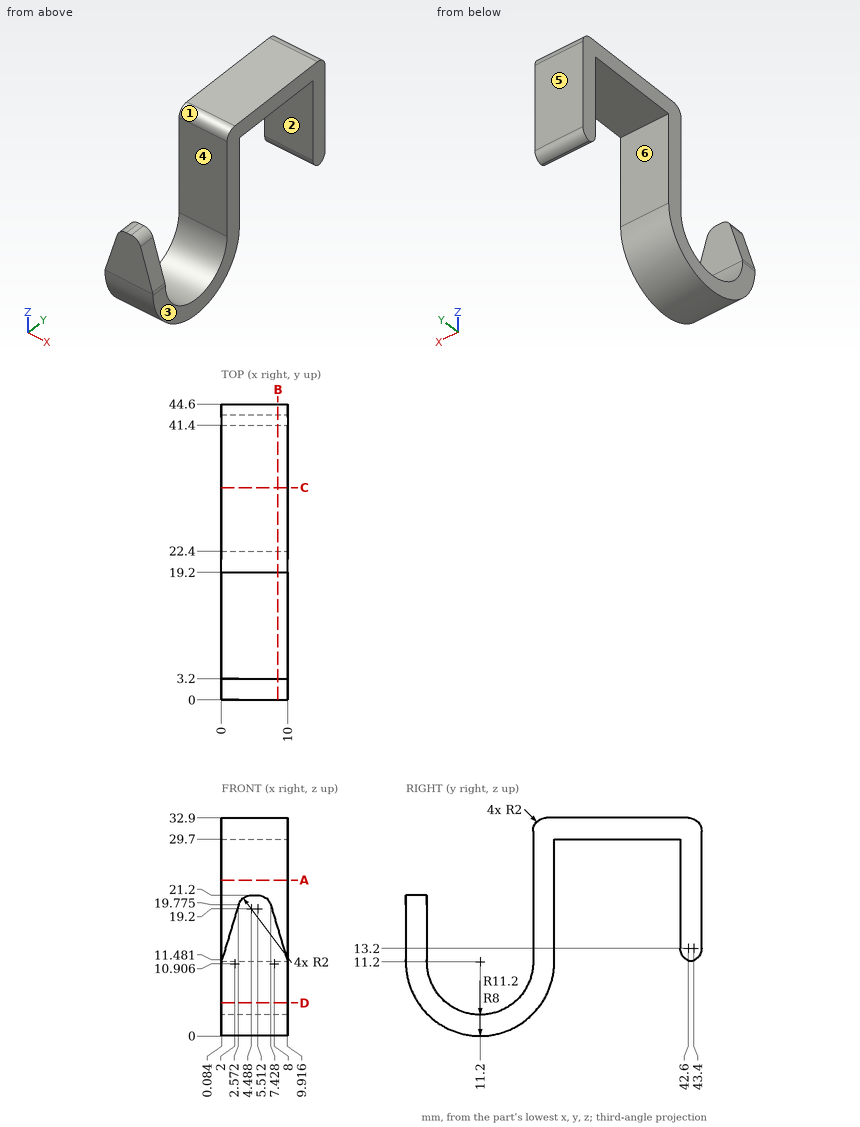
Part print with two shaded views. Sizes in mm from the minimum x, y, z corner. A direction names the side the tool comes from. Round coordinates to 2 decimals unless told otherwise and drop trailing zeros. Write each loop counter-clockwise with the first axis right and the second up, starting at its lowest first coordinate (ties: lowest second). Pieces come first, ordered by that corner, then holes. Notation, with made-up numbers: M -20,28 L -9,28 A27 cw -9,65 Z; hole C 49,67.5 d2. An arc over 180 degrees is marked long. Answer as CSV lines item,"result". Start each with the question number.
1) Drill centre lines: L1, parallel to Y at x = 4.5, z = 19; L2, parallel to Y at x = 1, z = 25.5; L3, parallel to Y at x = 9, z = 12. Where is each one in solid material? Low to high.
2) Band-saw the part on D-D (z = 5). List the corners of the cut face in (x, y) (1 decimal).
3) Band-saw the part on B-B (x = 8.5). List the corners of the cut face in (y, z).
4) Drop flat-ended pins along their axis: pin 1 (3 mm diameter, centred on x = 1.5, y = 6, fed in from -Z); pin 2 (2 mm diameter, centred on x = 4, y = 8, fed in from -Z); pin 3 (5 mm diameter, centred on x = 5.5, y = 9, fed in from +Z) (1 decimal). Give the stop position or say it passes through.
5) Which spindle directions (+Z, -Z, +X, -X, +Y, -Y) get a long thin tool onto all of the face, cutting with end or side? Do the marked faces 4, 5 and 6. Say none if no direction does.
6) Band-saw the part on C-C (y = 32). List the corners of the cut face in (x, z).
7) Band-saw the part on A-A (z = 23.5). List the corners of the cut face in (x, y).
8) Mould opens along Y. For the marked faces 1, 2 and 3 say: +Y half, -Y half, draft (parallel to the pull), parting line (faces both ways), or undercut.
Worked out:
1,L1,"0 to 3.2, 19.2 to 22.4, 41.4 to 44.6"
1,L2,"19.2 to 22.4, 41.4 to 44.6"
1,L3,"0 to 3.2, 19.2 to 22.4, 41.8 to 44.2"
2,outline,"M 0,1.9 L 10,1.9 L 10,6.1 L 0,6.1 Z; M 0,16.3 L 10,16.3 L 10,20.5 L 0,20.5 Z"
3,outline,"M 0,11.2 A11.2 ccw 22.4,11.2 L 22.4,29.7 L 41.4,29.7 L 41.4,13.2 A2 ccw 43,11.24 A2 ccw 44.6,13.2 L 44.6,30.9 A2 ccw 42.6,32.9 L 21.2,32.9 A2 ccw 19.2,30.9 L 19.2,11.2 A8 cw 3.2,11.2 L 3.2,16.2 L 0,16.2 Z"
4,pin 1,"z = 0.63"
4,pin 2,"z = 0.22"
4,pin 3,"z = 4.7"
5,face 4,"+Z, +X, -X"
5,face 5,"+Z, -Z, +X, -X, +Y"
5,face 6,"-Z, +X, -X"
6,outline,"M 0,29.7 L 10,29.7 L 10,32.9 L 0,32.9 Z"
7,outline,"M 0,19.2 L 10,19.2 L 10,22.4 L 0,22.4 Z; M 0,41.4 L 10,41.4 L 10,44.6 L 0,44.6 Z"
8,face 1,"-Y half"
8,face 2,"undercut"
8,face 3,"draft"
